The drawing under review shows one solid part. Ordinate dimensions are in mm from its lowest x, y, z. A direction names the side the tool comes from. Coordinates: 2 decimals unless noted, no trailing zeros. Loops run counter-clockwise (first coordinate to the right, second up) from the corner with the lowest first, then second, coordinate; pieces in that order, holes last. Notation, with made-up numbers: M -1,-8.75 L 44,-8.75 A24 cw 44,3.25 Z; hole C 8,43.5 d4. An arc over 180 degrees is marked long. Answer as a JSON object with one key per item and string values. Group by question number.
1. Consider section A-A (x = 10). State the section outline as (y, z) points, then the cut area to 3 significant figures.
2. To check wall thickness, follow probe 1 along Y at (x, z) = (10, 1.7); probe 2 along Z at (x, y) = (4, 12.75); probe 3 along X at (y, z) = (9.5, 13). State the ranges of each line that lie inside material, in increasing order.
3. Consider section D-D (z = 14.5). State the section outline as (x, y) points, then the cut area to 3 significant figures.
4. Consider section B-B (y = 2.5). State the section outline as (x, z) points, then the cut area to 3 significant figures.
5. Insertion check: pin 1 (8 mm diameter, centred on x = 14, y = 17.5, fed in from +Z); pin 2 (4 mm diameter, centred on y = 3.5, z = 3.5, fed in from -X); pin 3 (8 mm diameter, centred on y = 6, z = 15, fed in from +X). Each pin has a flat end and moves straight along its axis. Give the tip position at first contact, or say it passes through.
6. Machinability: for the marked faces 1 and 2, which of the approach directions +Z, -Z, +X, -X, +Y, -Y give a long, thin tool a straight path to every point of the face, cutting with its end or side? Answer none if there is none.
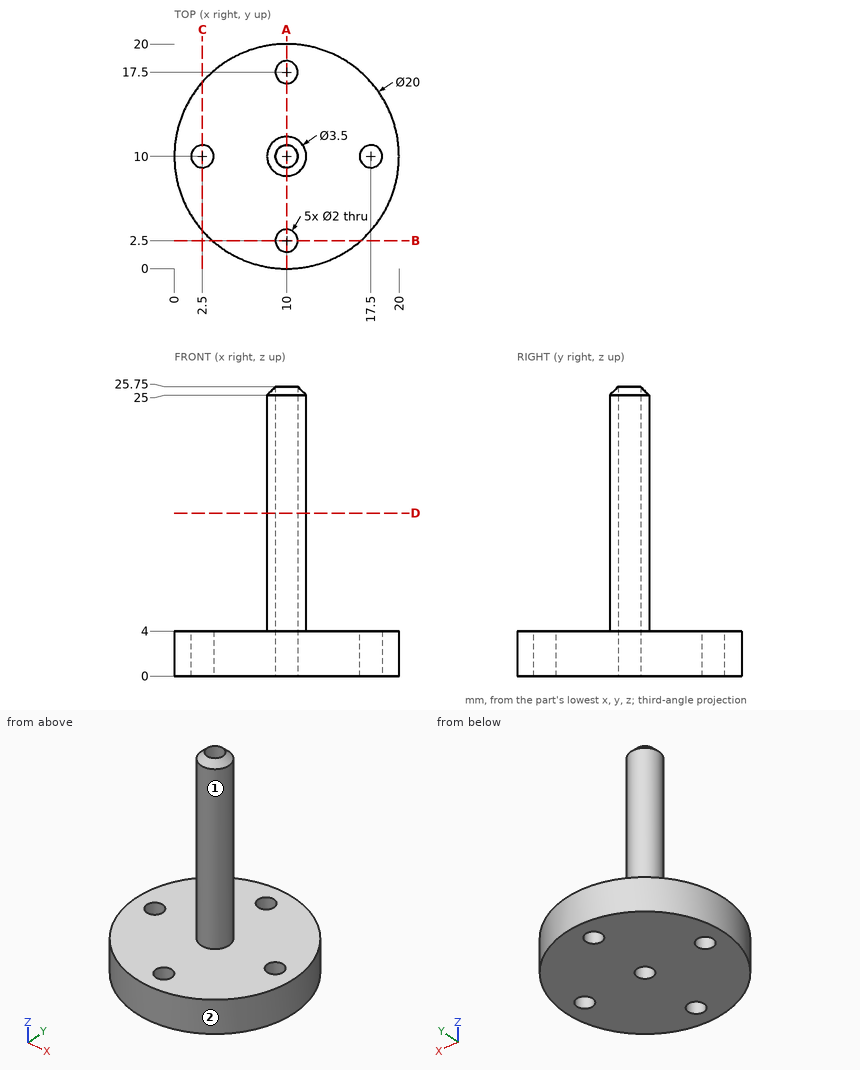
Findings below:
{
 "1": {"outline": "M 0,0 L 1.5,0 L 1.5,4 L 0,4 Z; M 3.5,0 L 9,0 L 9,25.75 L 8.25,25 L 8.25,4 L 3.5,4 Z; M 11,0 L 16.5,0 L 16.5,4 L 11.75,4 L 11.75,25 L 11,25.75 Z; M 18.5,0 L 20,0 L 20,4 L 18.5,4 Z", "area": "88.1 mm^2"},
 "2": {"probe 1": "y = 0 to 1.5, 3.5 to 9, 11 to 16.5, 18.5 to 20", "probe 2": "z = 0 to 4", "probe 3": "x = 8.32 to 9.13, 10.87 to 11.68"},
 "3": {"outline": "C 10,10 d3.5; hole C 10,10 d2", "area": "6.48 mm^2"},
 "4": {"outline": "M 3.39,0 L 9,0 L 9,4 L 3.39,4 Z; M 11,0 L 16.61,0 L 16.61,4 L 11,4 Z", "area": "44.9 mm^2"},
 "5": {"pin 1": "stops at z = 4", "pin 2": "stops at x = 1.07", "pin 3": "stops at x = 11.75"},
 "6": {"face 1": "+Z", "face 2": "+Z, -Z"}
}
